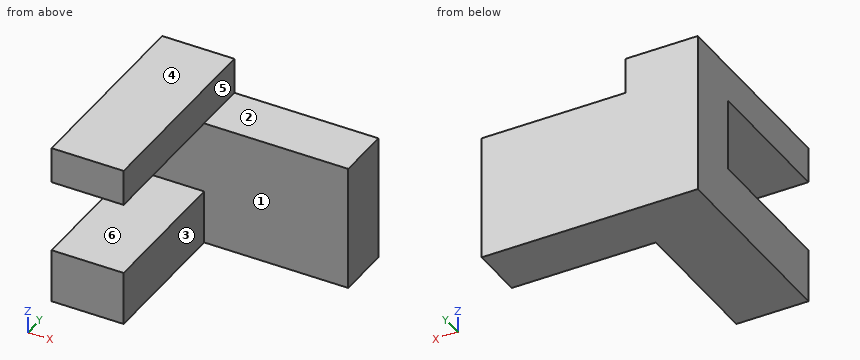
from build123d import *

# Parameters (mm, degrees)
F0_W     = 40
F0_H     = 15
F1_DEPTH = 60
F2_W     = 40
F2_H     = 40
F3_DEPTH = 45.001
F4_W     = 40
F4_H     = 10
F5_DEPTH = 25


with BuildPart() as f1:
    # F0 (on Right) → F1 (new body)
    with BuildSketch(Plane.YZ):
        Polygon((-15, 0), (0, 0), (0, 27.873229), (-15, 27.873229), (-15, 15), align=None)
        with Locations((-35, 7.5)):
            Rectangle(F0_W, F0_H)
        Polygon((-15, 27.873229), (0, 27.873229), (0, 45), (-55, 45), (-55, 35), (-15, 35), align=None)
    extrude(amount=F1_DEPTH)

    # F2 (on face) → F3 (cut, through all)
    with BuildSketch(Plane.XY.offset(45)):
        with Locations((40, -35)):
            Rectangle(F2_W, F2_H)
    extrude(amount=-F3_DEPTH, mode=Mode.SUBTRACT)

    # F4 (on face) → F5 (cut)
    with BuildSketch(Plane.XZ.offset(15)):
        with Locations((40, 40)):
            Rectangle(F4_W, F4_H)
    extrude(amount=-F5_DEPTH, mode=Mode.SUBTRACT)


solid = f1.part
Check sheet for the modelled part. Datum: model origin and axes. Units: mm. Face numbers are marked on the shaded views. A direction names the side the tool comes from. Give positions to 0.01 mm unless a question says otherwise; leave off trailing zeros. Loops run counter-clockwise (first coordinate to the right, second up) from the corner with the lowest first, then second, coordinate; pieces in that order, holes last. Notation, with made-up numbers: M 78.5,71 L 93.5,71 A27 ccw 93.5,87 Z; hole C -36.5,-8 d10. An arc over 180 degrees is marked long. Answer as a JSON object with one key per item and string values. Group by question number.
Q1. Material ranges on line 1 along Z through (x, y) = (15.5, -28.5); line 2 along Y through (x, z) = (49, 18.5); line 3 along Z through (x, y) = (38, -4), recorded low to high. Write a range as [from, to].
Q2. Cross-section at C-C on z = 8. Record the cut outline in (x, y).
Q3. Cross-section at D-D on y = -11. Record the cut outline in (x, z).
Q4. Cross-section at A-A on y = -36. Record the cut outline in (x, z).
Q5. Go/stop test with flat-tipped pins: P1, Ø16.5, axis at x = 44.5, y = -6.5, coming from the +Z side; P2, Ø3, axis at y = -33.5, z = 41, coming from the +X side; P3, Ø2, axis at y = -23.5, z = 33, coming from the +X side. Record where each tip stops, or that it passes through.
Q6. Cross-section at B-B on x = 9.5. Record the cut outline in (y, z), then the cut area to 4 significant figures.
Q7. Access from +Z, -Z, +X, -X, +Y, -Y to the whole of each face (thin tool, end or side, straight path). Record for the marked faces 4, 5 and 6.
Q8. Release check for a two-part mould opening along Z. For the marked faces 1, 2 and 3 record: released by +Z, released by -Z, zero draft, split by the parting line, or undercut.
Evaluation:
{
 "1": {"line 1": "z = [0, 15], [35, 45]", "line 2": "y = [-15, 0]", "line 3": "z = [0, 35]"},
 "2": {"outline": "M 0,-55 L 20,-55 L 20,-15 L 60,-15 L 60,0 L 0,0 Z"},
 "3": {"outline": "M 0,0 L 60,0 L 60,35 L 20,35 L 20,45 L 0,45 Z"},
 "4": {"outline": "M 0,0 L 20,0 L 20,15 L 0,15 Z; M 0,35 L 20,35 L 20,45 L 0,45 Z"},
 "5": {"P1": "stops at z = 35", "P2": "stops at x = 20", "P3": "passes through"},
 "6": {"outline": "M -55,0 L 0,0 L 0,45 L -55,45 L -55,35 L -15,35 L -15,15 L -55,15 Z", "area": "1,675 mm2"},
 "7": {"face 4": "+Z, +X, -X, +Y, -Y", "face 5": "+Z, +X, +Y, -Y", "face 6": "+X, -X, -Y"},
 "8": {"face 1": "undercut", "face 2": "released by +Z", "face 3": "zero draft"}
}
